from build123d import *

# Parameters (mm, degrees)
RESSALTO_EXTRUS_O1_DEPTH = 10
ESBO_O2_W                = 10
ESBO_O2_H                = 10
ESBO_O2_W_2              = 210
ESBO_O2_H_2              = 220
RESSALTO_EXTRUS_O4_DEPTH = 70
ESBO_O7_R                = 40
CORTE_EXTRUS_O1_DEPTH    = 3
ESBO_O21_W               = 200
ESBO_O21_H               = 45
CORTE_EXTRUS_O5_DEPTH    = 100
RESSALTO_EXTRUS_O5_DEPTH = 80
ESBO_O29_W               = 110
ESBO_O29_H               = 80
CORTE_EXTRUS_O8_DEPTH    = 250
ESBO_O30_W               = 12
ESBO_O30_H               = 10
RESSALTO_EXTRUS_O6_DEPTH = 50
ESBO_O31_W               = 100
ESBO_O31_H               = 90
CORTE_EXTRUS_O9_DEPTH    = 70
ESBO_O38_W               = 12
ESBO_O38_H               = 70
RESSALTO_EXTRUS_O8_DEPTH = 220
ESBO_O39_W               = 10
ESBO_O39_H               = 10
ESBO_O39_W_2             = 12
CORTE_EXTRUS_O10_DEPTH   = 10
ESBO_O40_W               = 88
ESBO_O40_H               = 10
CORTE_EXTRUS_O11_DEPTH   = 10


with BuildPart() as part:
    # Esboço1 → Ressalto-extrusão1 (new body)
    with BuildSketch(Plane.XY):
        Polygon((-99.217703787, 25.02394247), (70.782296213, 25.02394247), (70.782296213, 0), (70.782296213, -214.97605753), (-99.217703787, -214.97605753), (-269.217703787, -214.97605753), (-269.217703787, 0), (-269.217703787, 25.02394247), align=None)
    extrude(amount=RESSALTO_EXTRUS_O1_DEPTH)

    # Esboço2 → Ressalto-extrusão4 (add)
    with BuildSketch(Plane.XY.offset(10)):
        with Locations((-54.217703787, -209.97605753)):
            Rectangle(ESBO_O2_W, ESBO_O2_H)
        with Locations((-164.217703787, -209.97605753)):
            Rectangle(ESBO_O2_W_2, ESBO_O2_H)
        with Locations((-54.217703787, -94.97605753)):
            Rectangle(ESBO_O2_W, ESBO_O2_H_2)
        Polygon((-59.217703787, 15.02394247), (-49.217703787, 15.02394247), (-49.217703787, 25.02394247), (-269.217703787, 25.02394247), (-269.217703787, 15.02394247), align=None)
    extrude(amount=RESSALTO_EXTRUS_O4_DEPTH)

    # Esboço7 → Corte-extrusão1 (cut)
    with BuildSketch(Plane.XY.offset(10)):
        with Locations((10.782296213, -154.97605753)):
            Circle(ESBO_O7_R)
    extrude(amount=-CORTE_EXTRUS_O1_DEPTH, mode=Mode.SUBTRACT)

    # Esboço21 → Corte-extrusão5 (cut)
    with BuildSketch(Plane(origin=(0, 25.02394247, 0), x_dir=(1, 0, 0), z_dir=(0, 1, 0))):
        with Locations((-159.217703787, -47.5)):
            Rectangle(ESBO_O21_W, ESBO_O21_H)
    extrude(amount=-CORTE_EXTRUS_O5_DEPTH, mode=Mode.SUBTRACT)

    # Esboço28 → Ressalto-extrusão5 (add)
    with BuildSketch(Plane.XY.offset(10)):
        Polygon((70.782296213, -84.97605753), (70.782296213, 25.02394247), (60.782296213, 25.02394247), (-39.217703787, 25.02394247), (-49.217703787, 25.02394247), (-49.217703787, -74.97605753), (-49.217703787, -84.97605753), align=None)
    extrude(amount=RESSALTO_EXTRUS_O5_DEPTH)

    # Esboço29 → Corte-extrusão8 (cut)
    with BuildSketch(Plane.XZ.offset(214.97605753)):
        with Locations((-214.217703787, 40)):
            Rectangle(ESBO_O29_W, ESBO_O29_H)
    extrude(amount=-CORTE_EXTRUS_O8_DEPTH, mode=Mode.SUBTRACT)

    # Esboço30 → Ressalto-extrusão6 (add)
    with BuildSketch(Plane.XY.offset(25)):
        with Locations((-153.217703787, 20.02394247)):
            Rectangle(ESBO_O30_W, ESBO_O30_H)
    extrude(amount=RESSALTO_EXTRUS_O6_DEPTH)

    # Esboço31 → Corte-extrusão9 (cut)
    with BuildSketch(Plane.XY.offset(90)):
        with Locations((10.782296213, -29.97605753)):
            Rectangle(ESBO_O31_W, ESBO_O31_H)
    extrude(amount=-CORTE_EXTRUS_O9_DEPTH, mode=Mode.SUBTRACT)

    # Esboço38 → Ressalto-extrusão8 (add)
    with BuildSketch(Plane.XZ.offset(-15.02394247)):
        with Locations((-153.217703787, 45)):
            Rectangle(ESBO_O38_W, ESBO_O38_H)
    extrude(amount=RESSALTO_EXTRUS_O8_DEPTH)

    # Esboço39 → Corte-extrusão10 (cut)
    with BuildSketch(Plane.XY.offset(80)):
        with Locations((-54.217703787, -94.97605753)):
            Rectangle(ESBO_O39_W, ESBO_O39_H)
        with Locations((-153.217703787, -94.97605753)):
            Rectangle(ESBO_O39_W_2, ESBO_O39_H)
    extrude(amount=-CORTE_EXTRUS_O10_DEPTH, mode=Mode.SUBTRACT)

    # Esboço40 → Corte-extrusão11 (cut)
    with BuildSketch(Plane(origin=(0, 25.02394247, 0), x_dir=(1, 0, 0), z_dir=(0, 1, 0))):
        with Locations((-103.217703787, -75)):
            Rectangle(ESBO_O40_W, ESBO_O40_H)
    extrude(amount=-CORTE_EXTRUS_O11_DEPTH, mode=Mode.SUBTRACT)


solid = part.part
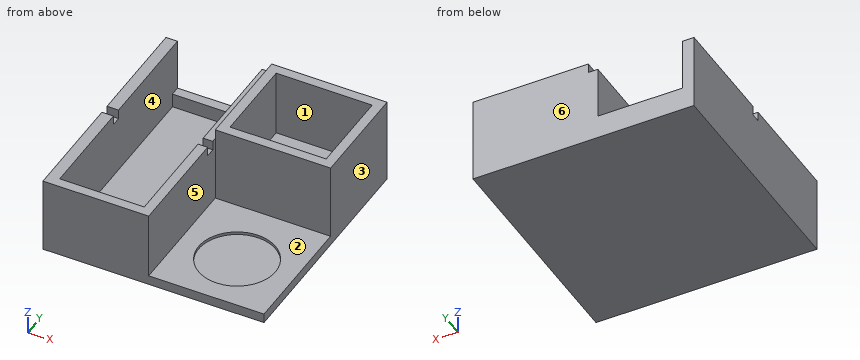
Could you check a few things on this model? Use its own coordinates, in mm. Face numbers are marked on the shaded views. A direction names the side the tool comes from. Coordinates: 2 decimals unless noted, no trailing zeros. Order: outer loops, then holes, each group sorted by start corner. A loop starts at its lowest first (then second) coordinate and runs counter-clockwise, first axis right, second up.
Q1. Suppose I cut it at C-C on y = -79. Please give me the cut outline in (x, z), and give its area (3 significant figures).
Q2. Suppose I cut it at B-B on x = -62. Please give me the cut outline in (y, z), and give its area (3 significant figures).
Q3. Which directions (+Z, -Z, +X, -X, +Y, -Y) give clear straight access to the entire face, cutting with the end or side of a thin tool? Please do the marked faces 1, 2 and 3.
Q4. Suppose I cut it at A-A on z = 77. Please give me the cut outline in (x, y), and give its area (3 significant figures).
Q5. Please list where these lines run through material, in increasing order: L1, parallel to X at y = -30, z = 25; L2, parallel to X at y = -19, z = 10.5; L3, parallel to Y at x = 15.5, z = 54.
Q6. Suppose I cut it at D-D on y = -3. Please give me the cut outline in (x, z).
Q7. Will these pins go through, and if not, where does the flat tip stop? pin 1 (12 mm diameter, centred on x = -58, y = -175, fed in from +Z); pin 2 (3 mm diameter, centred on x = -67, y = -35, fed in from +Z); pin 3 (5 mm diameter, centred on x = -153, y = -94.5, fed in from +Z).
Q8. Thinking about a two-plate mould opening in Y: for the marked faces 4, 5 and 6, which applies, released by +Y, released by -Y, zero draft, split by the parting line, or undercut?
Answer:
1. outline: (-159.22, 0) - (70.78, 0) - (70.78, 90) - (-49.22, 90) - (-49.22, 80) - (-59.22, 80) - (-59.22, 10) - (-147.22, 10) - (-147.22, 80) - (-159.22, 80) - close
1. area: 13,400 mm2
2. outline: (-214.98, 0) - (25.02, 0) - (25.02, 25) - (15.02, 25) - (15.02, 10) - (-204.98, 10) - (-204.98, 80) - (-214.98, 80) - close
2. area: 3,250 mm2
3. face 1: +Z
3. face 2: +Z, +X, -Y
3. face 3: +Z, -Z, +X, +Y, -Y
4. outline: (-159.22, -214.98) - (-49.22, -214.98) - (-49.22, -99.98) - (-59.22, -99.98) - (-59.22, -204.98) - (-147.22, -204.98) - (-147.22, -99.98) - (-159.22, -99.98) - close; (-159.22, -89.98) - (-147.22, -89.98) - (-147.22, 25.02) - (-159.22, 25.02) - close; (-59.22, -89.98) - (-49.22, -89.98) - (-49.22, -84.98) - (70.78, -84.98) - (70.78, 25.02) - (-59.22, 25.02) - close; hole (-39.22, -74.98) - (60.78, -74.98) - (60.78, 15.02) - (-39.22, 15.02) - close
4. area: 10,100 mm2
5. L1: x = -159.22 to -147.22, -59.22 to -39.22, 60.78 to 70.78
5. L2: x = -159.22 to -147.22, -59.22 to 70.78
5. L3: y = -84.98 to -74.98, 15.02 to 25.02
6. outline: (-159.22, 0) - (70.78, 0) - (70.78, 90) - (60.78, 90) - (60.78, 20) - (-39.22, 20) - (-39.22, 90) - (-49.22, 90) - (-49.22, 80) - (-59.22, 80) - (-59.22, 10) - (-147.22, 10) - (-147.22, 80) - (-159.22, 80) - close
7. pin 1: stops at z = 80
7. pin 2: stops at z = 10
7. pin 3: stops at z = 70
8. face 4: undercut
8. face 5: zero draft
8. face 6: released by +Y
